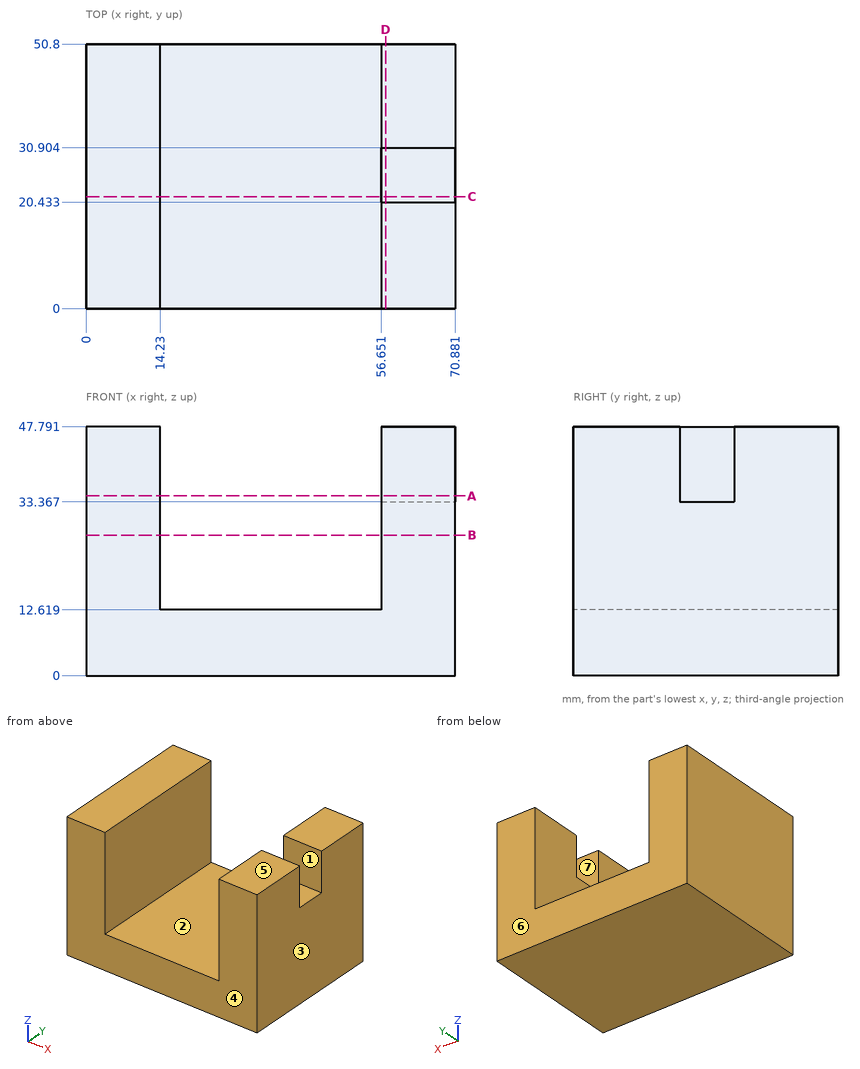
The figure shows three views and two pictorial views of one solid part (mm, origin at its lowest corner). Answer the questions. A direction names the side the tool comes from. Coordinates: 2 decimals unless noted, no trailing zeros. Write each loop counter-clockwise with the first axis right and the second up, starting at its lowest first coordinate (ties: lowest second). Pieces come first, ordered by that corner, then holes. Notation, with made-up numbers: (-24.5, 49.5) -> (-20.5, 49.5) arc R25 cw to (-20.5, 79.5) -> close; hole circle Ø1 at (62, 84.25). An arc over 180 degrees is marked (long way). Return JSON: item names as keys, results as strings.
1. Determine the mould class of the marked faces 4, 5, 6 and 7 for opening direction Y: pulls with the +Y half, pulls with the -Y half, needs draft (parallel to the pull), parting line crosses it, or undercut.
Found:
{"face 4": "pulls with the -Y half", "face 5": "needs draft", "face 6": "pulls with the +Y half", "face 7": "undercut"}
2. Each of these flat-tipped pins is pushed along its axis until it touches: P1, Ø4, axis at y = 14.5, z = 41, coming from the -X side; P2, Ø5, axis at x = 26, y = 8, coming from the +Z side; P3, Ø5, axis at x = 66, y = 26.5, coming from the +Z side; P4, Ø1.5, axis at y = 24.5, z = 34.5, coming from the +X side. Where does it stop, or does it pass through?
Found:
{"P1": "x = 0", "P2": "z = 12.62", "P3": "z = 33.37", "P4": "x = 14.23"}
3. A cutting plane is placed at C-C (y = 21.5). Determine the outline of the cut face in (x, z).
Found:
{"outline": "(0, 0) -> (70.88, 0) -> (70.88, 33.37) -> (56.65, 33.37) -> (56.65, 12.62) -> (14.23, 12.62) -> (14.23, 47.79) -> (0, 47.79) -> close"}
4. A cutting plane is placed at B-B (z = 27). Determine the outline of the cut face in (x, y), and give its area (3 significant figures).
Found:
{"outline": "(0, 0) -> (14.23, 0) -> (14.23, 50.8) -> (0, 50.8) -> close; (56.65, 0) -> (70.88, 0) -> (70.88, 50.8) -> (56.65, 50.8) -> close", "area": "1,450 mm2"}
5. A tool of negligible diameter and unlimited length cuts with its end or side. For the marked faces 1, 2 and 3, from which of +Z, -Z, +X, -X, +Y, -Y can it reach the whole face along a straight path? Write none if from no direction.
Found:
{"face 1": "+Z, +X", "face 2": "+Z, +Y, -Y", "face 3": "+Z, -Z, +X, +Y, -Y"}
6. Find the intervals of material crossed by line 1 along X through (y, z) = (17.5, 25.5); line 2 along Y through (x, z) = (67, 39.5); line 3 along Z through (x, y) = (20, 46.5), in increasing order. Write a range as from..to.
Found:
{"line 1": "0..14.23, 56.65..70.88", "line 2": "0..20.43, 30.9..50.8", "line 3": "0..12.62"}
7. A cutting plane is placed at D-D (x = 57.5). Determine the outline of the cut face in (y, z), and give its area (3 significant figures).
Found:
{"outline": "(0, 0) -> (50.8, 0) -> (50.8, 47.79) -> (30.9, 47.79) -> (30.9, 33.37) -> (20.43, 33.37) -> (20.43, 47.79) -> (0, 47.79) -> close", "area": "2,280 mm2"}
8. A cutting plane is placed at A-A (z = 34.5). Determine the outline of the cut face in (x, y), and give its area (3 significant figures).
Found:
{"outline": "(0, 0) -> (14.23, 0) -> (14.23, 50.8) -> (0, 50.8) -> close; (56.65, 0) -> (70.88, 0) -> (70.88, 20.43) -> (56.65, 20.43) -> close; (56.65, 30.9) -> (70.88, 30.9) -> (70.88, 50.8) -> (56.65, 50.8) -> close", "area": "1,300 mm2"}
